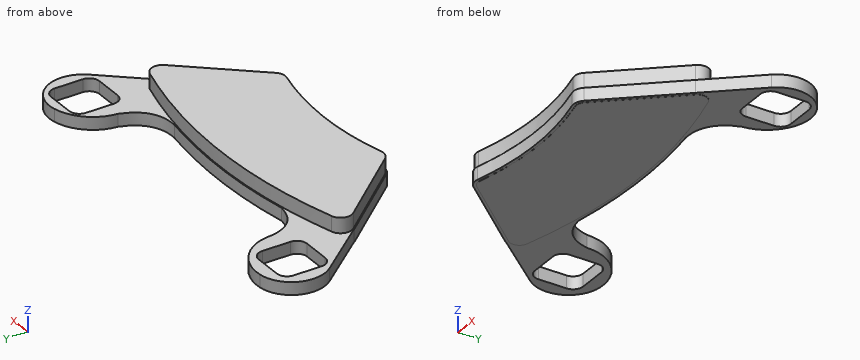
```python
from build123d import *

# Parameters (mm, degrees)
BOSS_EXTRUDE1_DEPTH = 3.429
FILLET1_R           = 2.54
BOSS_EXTRUDE2_DEPTH = 2.8448
BOSS_EXTRUDE3_DEPTH = 2.8448
FILLET2_R           = 7.62
CUT_EXTRUDE1_DEPTH  = 2.8448
BOSS_EXTRUDE4_DEPTH = 2.8448
CUT_EXTRUDE2_DEPTH  = 2.8448
FILLET3_R           = 7.62
BOSS_EXTRUDE5_DEPTH = 0.0254


with BuildPart() as part:
    # Sketch1 → Boss-Extrude1 (new body)
    with BuildSketch(Plane.XY):
        with BuildLine():
            Line((-35.365163415, 20.32), (-17.839163415, 0))
            add(Edge.make_bspline(
                [(-17.839163415, 0), (0.211689908, 5.080726576), (18.279636585, 0)],
                knots=[0, 0, 0, 1, 1, 1], degree=2))
            Line((18.279636585, 0), (35.805636585, 20.32))
            add(Edge.make_bspline(
                [(-35.365163415, 20.32), (0.209256434, 31.699614416), (35.805636585, 20.32)],
                knots=[0, 0, 0, 1, 1, 1], degree=2))
        make_face()
    extrude(amount=BOSS_EXTRUDE1_DEPTH)

    # Fillet1
    fillet1_edges = [part.edges().sort_by_distance(p)[0] for p in [
        (18.279636585, 0, 1.7145),
        (35.805636585, 20.32, 1.7145),
        (-17.839163415, 0, 1.7145),
        (-35.365163415, 20.32, 1.7145),
    ]]
    fillet(fillet1_edges, radius=FILLET1_R)

    # Sketch3 → Boss-Extrude2 (add)
    with BuildSketch(Plane(origin=(0, 0, 0), x_dir=(-1, 0, 0), z_dir=(0, 0, -1))):
        with BuildLine():
            Line((-33.44681638, 17.196237572), (-19.51455408, 1.042889978))
            ThreePointArc((-19.51455408, 1.042889978), (-18.233735028, 0.201395136), (-16.701721503, 0.162081334))
            add(Edge.make_bspline(
                [(-16.701721503, 0.162081334), (-11.287416328, 1.557018557), (-5.815998288, 2.280480011), (1.099570731, 2.287789464), (2.486501294, 2.244377729), (5.268126494, 2.066272068), (6.66342146, 1.931190975), (10.814897092, 1.394504939), (13.552184291, 0.860935066), (16.260993662, 0.162500978)],
                knots=[0, 0, 0, 0, 0.5, 0.5, 0.625, 0.625, 0.75, 0.75, 1, 1, 1, 1], degree=3))
            ThreePointArc((16.260993662, 0.162500978), (17.793263077, 0.201606931), (19.074330708, 1.043179601))
            Line((19.074330708, 1.043179601), (33.006779663, 17.196743606))
            ThreePointArc((33.006779663, 17.196743606), (33.568121111, 19.821332934), (31.659110958, 21.707931354))
            add(Edge.make_bspline(
                [(31.659110958, 21.707931354), (21.234977833, 24.688407586), (10.651761037, 26.253278411), (-1.450873571, 26.265063816), (-2.798343422, 26.242056629), (-5.498815234, 26.146814801), (-6.854115547, 26.074394022), (-10.909317669, 25.783877715), (-13.59595314, 25.493149433), (-21.607199162, 24.340406402), (-26.883182271, 23.198023422), (-32.098788298, 21.707528048)],
                knots=[0, 0, 0, 0, 0.5, 0.5, 0.5625, 0.5625, 0.625, 0.625, 0.75, 0.75, 1, 1, 1, 1], degree=3))
            ThreePointArc((-32.098788298, 21.707528048), (-34.008104328, 19.821005964), (-33.44681638, 17.196237572))
        make_face()
    extrude(amount=BOSS_EXTRUDE2_DEPTH)

    # Sketch6 → Boss-Extrude3 (add)
    with BuildSketch(Plane(origin=(0, 0, -2.8448), x_dir=(-1, 0, 0), z_dir=(0, 0, -1))):
        with BuildLine():
            Line((18.860011299, 24.632736939), (22.773121111, 23.894535093))
            Line((22.773121111, 23.894535093), (30.902144608, 14.756587021))
            Line((30.902144608, 14.756587021), (46.651415509, 33.752843138))
            ThreePointArc((46.651415509, 33.752843138), (35.612340647, 41.602210449), (26.583121111, 31.505332934))
            add(Edge.make_bspline(
                [(26.583121111, 31.505332934), (25.303985062, 25.198624265), (18.860011299, 24.632736939)],
                knots=[0, 0, 0, 1, 1, 1], degree=2))
        make_face()
    extrude(amount=-BOSS_EXTRUDE3_DEPTH)

    # Fillet2
    fillet2_edges = [part.edges().sort_by_distance(p)[0] for p in [
        (-46.651415509, 33.752843138, -1.4224),
    ]]
    fillet(fillet2_edges, radius=FILLET2_R)

    # Sketch8 → Cut-Extrude1 (cut)
    with BuildSketch(Plane(origin=(0, 0, -2.8448), x_dir=(-1, 0, 0), z_dir=(0, 0, -1))):
        with BuildLine():
            Line((32.846126677, 38.744332934), (39.196126677, 38.744332934))
            ThreePointArc((39.196126677, 38.744332934), (40.812572779, 38.074779036), (41.482126677, 36.458332934))
            Line((41.482126677, 36.458332934), (41.482126677, 30.108332934))
            ThreePointArc((41.482126677, 30.108332934), (40.812572779, 28.491886832), (39.196126677, 27.822332934))
            Line((39.196126677, 27.822332934), (32.846126677, 27.822332934))
            ThreePointArc((32.846126677, 27.822332934), (31.229680575, 28.491886832), (30.560126677, 30.108332934))
            Line((30.560126677, 30.108332934), (30.560126677, 36.458332934))
            ThreePointArc((30.560126677, 36.458332934), (31.229680575, 38.074779036), (32.846126677, 38.744332934))
        make_face()
    extrude(amount=-CUT_EXTRUDE1_DEPTH, mode=Mode.SUBTRACT)

    # Sketch9 → Boss-Extrude4 (add)
    with BuildSketch(Plane(origin=(0, 0, -2.8448), x_dir=(-1, 0, 0), z_dir=(0, 0, -1))):
        with BuildLine():
            Line((-47.463840908, 33.447860213), (-33.44681638, 17.196237572))
            Line((-33.44681638, 17.196237572), (-23.253298607, 23.884814358))
            Line((-23.253298607, 23.884814358), (-18.292818846, 24.798887742))
            add(Edge.make_bspline(
                [(-27.552629507, 31.505332934), (-25.268328972, 24.405957798), (-18.292818846, 24.798887742)],
                knots=[0, 0, 0, 1, 1, 1], degree=2))
            ThreePointArc((-27.552629507, 31.505332934), (-36.694543436, 40.817065736), (-47.463840908, 33.447860213))
        make_face()
    extrude(amount=-BOSS_EXTRUDE4_DEPTH)

    # Sketch10 → Cut-Extrude2 (cut)
    with BuildSketch(Plane(origin=(0, 0, -2.8448), x_dir=(-1, 0, 0), z_dir=(0, 0, -1))):
        with BuildLine():
            Line((-39.797873323, 38.744332934), (-33.447873323, 38.744332934))
            ThreePointArc((-33.447873323, 38.744332934), (-31.831427221, 38.074779036), (-31.161873323, 36.458332934))
            Line((-31.161873323, 36.458332934), (-31.161873323, 30.108332934))
            ThreePointArc((-31.161873323, 30.108332934), (-31.831427221, 28.491886832), (-33.447873323, 27.822332934))
            Line((-33.447873323, 27.822332934), (-39.797873323, 27.822332934))
            ThreePointArc((-39.797873323, 27.822332934), (-41.414319425, 28.491886832), (-42.083873323, 30.108332934))
            Line((-42.083873323, 30.108332934), (-42.083873323, 36.458332934))
            ThreePointArc((-42.083873323, 36.458332934), (-41.414319425, 38.074779036), (-39.797873323, 38.744332934))
        make_face()
    extrude(amount=-CUT_EXTRUDE2_DEPTH, mode=Mode.SUBTRACT)

    # Fillet3
    fillet3_edges = [part.edges().sort_by_distance(p)[0] for p in [
        (47.463840908, 33.447860213, -1.4224),
    ]]
    fillet(fillet3_edges, radius=FILLET3_R)

    # Sketch11 → Boss-Extrude5 (add)
    with BuildSketch(Plane(origin=(0, 0, -2.8448), x_dir=(-1, 0, 0), z_dir=(0, 0, -1))):
        with BuildLine():
            Line((-32.96596357, 17.610973121), (-19.03370127, 1.457625527))
            ThreePointArc((-19.03370127, 1.457625527), (-18.043977457, 0.807379512), (-16.860148825, 0.777000665))
            add(Edge.make_bspline(
                [(-16.860148825, 0.777000665), (-11.393767532, 2.185354737), (-5.869704309, 2.915437473), (1.112358732, 2.922799867), (2.512622955, 2.878981915), (5.320986764, 2.699211385), (6.729692814, 2.562868028), (10.921080204, 2.021141726), (13.684690054, 1.482537974), (16.419535692, 0.777390745)],
                knots=[0, 0, 0, 0, 0.5, 0.5, 0.625, 0.625, 0.75, 0.75, 1, 1, 1, 1], degree=3))
            ThreePointArc((16.419535692, 0.777390745), (17.603562029, 0.807609004), (18.593477899, 1.457915149))
            Line((18.593477899, 1.457915149), (32.525926853, 17.611479154))
            ThreePointArc((32.525926853, 17.611479154), (32.9596907, 19.639570906), (31.484546495, 21.097396958))
            add(Edge.make_bspline(
                [(31.484546495, 21.097396958), (21.117495606, 24.061552194), (10.592269896, 25.618335787), (-1.444129852, 25.63005698), (-2.78422621, 25.607170327), (-5.469922522, 25.512428381), (-6.817808951, 25.44038787), (-10.850823746, 25.151400244), (-13.522755051, 24.862204706), (-21.490147902, 23.715583367), (-26.737240722, 22.579309276), (-31.924305501, 21.096970308)],
                knots=[0, 0, 0, 0, 0.5, 0.5, 0.5625, 0.5625, 0.625, 0.625, 0.75, 0.75, 1, 1, 1, 1], degree=3))
            ThreePointArc((-31.924305501, 21.096970308), (-33.399686074, 19.639203245), (-32.96596357, 17.610973121))
        make_face()
    extrude(amount=BOSS_EXTRUDE5_DEPTH)


solid = part.part
```
The model under review builds one solid part; all positions refer to its coordinate system, in mm. Coordinates: 2 decimals unless noted, no trailing zeros. Write each loop counter-clockwise with the first axis right and the second up, starting at its lowest first coordinate (ties: lowest second). Pieces come first, ordered by that corner, then holes. Notation, with made-up numbers: (61, -10.5) - (90, -10.5) arc R10 ccw to (90, 5.5) - close; hole circle Ø5 at (7, 51.25). An arc over 180 degrees is marked (long way). Write item = value, one per line.
(1) Consider section C-C, the plane z = -2. State how many separate pieces and enclosed holes the cut face has, then the cut area to 3 significant figures.
Result sheet:
separate_pieces = 1
enclosed_holes = 2
area = 1,700 mm^2
(2) Consider section A-A, the plane y = 35. Give the boundary of the cut face in (x, z), then the cut area to 3 significant figures.
Result sheet:
outline = (-44.54, -2.84) - (-41.48, -2.84) - (-41.48, 0) - (-44.54, 0) - close; (-30.56, -2.84) - (-27.2, -2.84) - (-27.2, 0) - (-30.56, 0) - close; (28.47, -2.84) - (31.16, -2.84) - (31.16, 0) - (28.47, 0) - close; (42.08, -2.84) - (44.59, -2.84) - (44.59, 0) - (42.08, 0) - close
area = 33.0 mm^2
(3) For line 1 (Z direction, x = -29, y = 25); line 2 (X direction, y = 29, z = -2.5); line 3 (X direction, y = 19, z = 2), list the stretches that pass through material, from the lowest coordinate up. Write a range as [from, to].
Result sheet:
line_1 = [-2.84, 0]
line_2 = [-42.71, -41.2], [-30.85, -25.77], [26.47, 31.45], [41.8, 43.54]
line_3 = [-33.43, 33.87]
(4) For P1, Ø0.9, axis at x = -36, z = -2, coming from the +Y side; P2, Ø3, axis at x = 37, z = -1.5, coming from the +Y side; P3, Ø3, axis at y = 34.5, z = -2, coming from the -X side; P4, Ø2.5, axis at x = 37, z = -2, coming from the -Y side, all flat-tipped, find the tip position at first contact; note any pin that passes through.
Result sheet:
P1 = 41.66
P2 = 40.82
P3 = -44.61
P4 = 19.87
